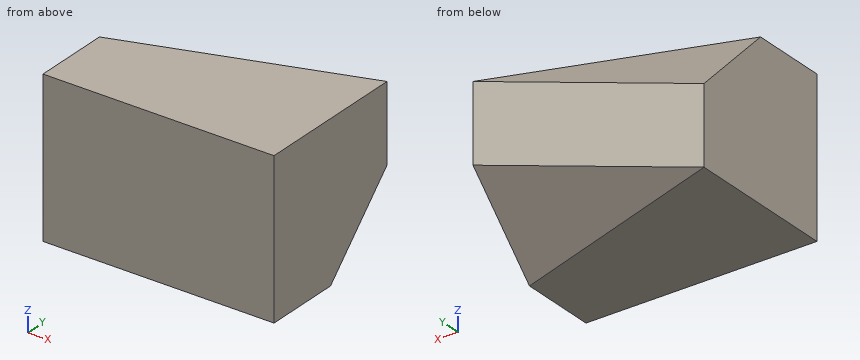
```python
from build123d import *

# Parameters (mm, degrees)
SKETCH_1_W          = 6
SKETCH_1_H          = 4
EXTRUDE_1_DEPTH     = 4
CUT_EXTRUDE_1_DEPTH = 4
SKETCH_10_W         = 32.252295377
SKETCH_10_H         = 15.179180951
CUT_EXTRUDE_2_DEPTH = 5


with BuildPart() as part:
    # 草圖1 → 填料-伸長1 (new body)
    with BuildSketch(Plane(origin=(0, 0, 0), x_dir=(1, 0, 0), z_dir=(0, 1, 0))):
        Rectangle(SKETCH_1_W, SKETCH_1_H)
    extrude(amount=EXTRUDE_1_DEPTH)

    # 草圖6 → 除料-伸長1 (cut)
    with BuildSketch(Plane(origin=(0.789473684, 2.368421053, -2.368421053), x_dir=(0.973328527, -0.162221421, 0.162221421), z_dir=(-0.229415734, -0.688247202, 0.688247202))):
        Polygon((0, 0), (-20.538761547, 0), (-20.538761547, 12.535207186), (11.71353383, 14.625633738), (12.268136792, -0.263322726), align=None)
    extrude(amount=-CUT_EXTRUDE_1_DEPTH, mode=Mode.SUBTRACT)

    # 草圖10 → 除料-伸長2 (cut)
    with BuildSketch(Plane(origin=(-0.789473684, 2.368421053, 2.368421053), x_dir=(0.973328527, 0.162221421, 0.162221421), z_dir=(-0.229415734, 0.688247202, 0.688247202))):
        with Locations((3.943334428, 7.114500239)):
            Rectangle(SKETCH_10_W, SKETCH_10_H)
    extrude(amount=CUT_EXTRUDE_2_DEPTH, mode=Mode.SUBTRACT)


solid = part.part
```
Check sheet for the modelled part. Datum: model origin and axes. Units: mm. Round coordinates to 2 decimals unless told otherwise and drop trailing zeros. Loops run counter-clockwise (first coordinate to the right, second up) from the corner with the lowest first, then second, coordinate; pieces in that order, holes last. Notation, with made-up numbers: (-13, 19) -> (6, 19) arc R7 cw to (6, 29) -> close; hole circle Ø8 at (86.5, 29). An arc over 180 degrees is marked (long way). Write item = value, one per line. Start each with the question number.
1) Sectioned sample at C-C, the plane x = 0. Record the cut outline in (y, z).
2) Sectioned sample at D-D, the plane z = -0.55. Record the cut outline in (x, y), plus the area to 3 significant figures.
3) Thickness scan on probe 1 along Z at (x, y) = (-2, 2.65); probe 2 along Y at (x, z) = (0, -1.05); probe 3 along Y at (x, z) = (-0.25, 1.4). Record the ranges inside material, lowest first.
4) Sectioned sample at A-A, the plane z = -1.3. Record the cut outline in (x, y), plus the area to 3 significant figures.
5) Sectioned sample at B-B, the plane y = 3.15. Record the cut outline in (x, z), plus the area to 3 significant figures.
Results are:
q1.outline = (0, -2) -> (3, -2) -> (4, -1) -> (4, 1) -> (3, 2) -> (0, 2) -> close
q2.outline = (-3, 0) -> (3, 0) -> (3, 3.45) -> (1.35, 4) -> (-3, 4) -> close
q2.area = 23.5 mm^2
q3.probe_1 = -2 to 1.68
q3.probe_2 = 0 to 3.95
q3.probe_3 = 0 to 3.52
q4.outline = (-3, 0) -> (3, 0) -> (3, 2.7) -> (-0.9, 4) -> (-3, 4) -> close
q4.area = 21.5 mm^2
q5.outline = (-3, -2) -> (-0.45, -2) -> (3, -0.85) -> (3, 2) -> (0.45, 2) -> (-3, 0.85) -> close
q5.area = 20.0 mm^2
